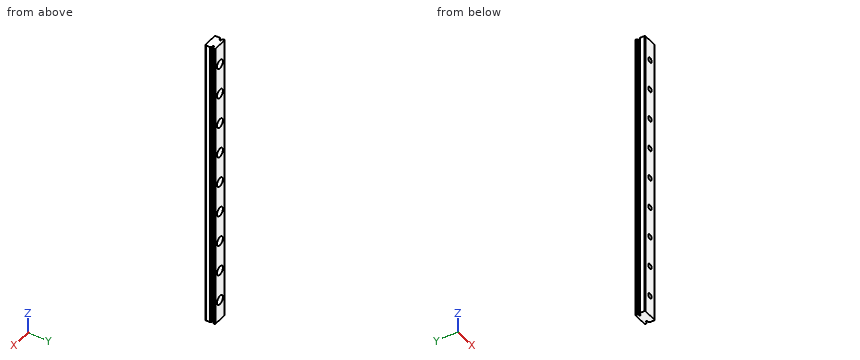
Autodesk Inventor part; units mm, degrees
ref_plane "to_block_XY" through (0, 4.7, 35) normal (0, 0, -1) x (1, 0, 0)
ref_plane "to_block_YZ" through (0, 4.7, 35) normal (1, 0, 0) x (0, -1, 0)
ref_plane "to_block_ZX" through (0, 4.7, 35) normal (0, -1, 0) x (0, 0, -1)
sketch "Sketch_12" plane through (0, 0, 0) normal (0, 0, 1) x (1, 0, 0)
  line L0 (-3.5, 4.4) -> (-3.5, 4.0339)
  line L1 (-3.5, 4.0339) -> (-3.2695, 3.9008)
  arc A0 (-2.9324, 3.55) -> (-3.2695, 3.9008) centre (-3.707, 3.143) ccw
  line L2 (-2.9324, 3.55) -> (-2.2, 3.55)
  line L3 (-2.2, 3.55) -> (-2.2, 2.85)
  line L4 (-2.2, 2.85) -> (-2.9324, 2.85)
  arc A1 (-3.2695, 2.4992) -> (-2.9324, 2.85) centre (-3.707, 3.257) ccw
  line L5 (-3.2695, 2.4992) -> (-3.5, 2.3662)
  line L6 (-3.5, 2.3662) -> (-3.5, 0.3)
  line L7 (-3.5, 0.3) -> (-3.2, 0)
  line L8 (-3.2, 0) -> (3.2, 0)
  line L9 (3.2, 0) -> (3.5, 0.3)
  line L10 (3.5, 0.3) -> (3.5, 2.3662)
  line L11 (3.5, 2.3662) -> (3.2695, 2.4992)
  arc A2 (2.9324, 2.85) -> (3.2695, 2.4992) centre (3.707, 3.257) ccw
  line L12 (2.9324, 2.85) -> (2.2, 2.85)
  line L13 (2.2, 2.85) -> (2.2, 3.55)
  line L14 (2.2, 3.55) -> (2.9324, 3.55)
  arc A3 (3.2695, 3.9008) -> (2.9324, 3.55) centre (3.707, 3.143) ccw
  line L15 (3.2695, 3.9008) -> (3.5, 4.0339)
  line L16 (3.5, 4.0339) -> (3.5, 4.4)
  line L17 (3.5, 4.4) -> (3.2, 4.7)
  line L18 (3.2, 4.7) -> (-3.2, 4.7)
  line L19 (-3.2, 4.7) -> (-3.5, 4.4)
extrude "Extrusion1" add sketch "Sketch_12" along normal mid plane 140
sketch "Sketch2" plane through (-3.2, 4.7, 70) normal (0, 1, 0) x (1, 0, 0)
  point P0 (3.2, 130)
hole "Hole1" at (0, 4.7, -60) direction (0, -1, 0) diameter 2.4 depth 4.7 counterbore diameter 4.2 counterbore depth 2.3
pattern_linear "Rectangular Pattern1" count 9 spacing 15 along (0, 0, 1) of "Hole1"
ref_plane "to_block_XY" through (0, 4.7, 35) normal (0, 0, -1) x (1, 0, 0)
ref_plane "to_block_YZ" through (0, 4.7, 35) normal (1, 0, 0) x (0, -1, 0)
ref_plane "to_block_ZX" through (0, 4.7, 35) normal (0, -1, 0) x (0, 0, -1)
ref_plane "to_block_2_XY" through (0, 4.7, -35) normal (0, 0, -1) x (1, 0, 0)
ref_plane "to_block_2_YZ" through (0, 4.7, -35) normal (1, 0, 0) x (0, -1, 0)
ref_plane "to_block_2_ZX" through (0, 4.7, -35) normal (0, -1, 0) x (0, 0, -1)
ref_plane "to_bolt_1_XY" through (0, 2.4, 60) normal (0, 1, 0) x (1, 0, 0)
ref_plane "to_bolt_1_YZ" through (0, 2.4, 60) normal (1, 0, 0) x (0, 0, -1)
ref_plane "to_bolt_1_ZX" through (0, 2.4, 60) normal (0, 0, -1) x (0, 1, 0)
ref_plane "to_bolt_2_XY" through (0, 2.4, 45) normal (0, 1, 0) x (1, 0, 0)
ref_plane "to_bolt_2_YZ" through (0, 2.4, 45) normal (1, 0, 0) x (0, 0, -1)
ref_plane "to_bolt_2_ZX" through (0, 2.4, 45) normal (0, 0, -1) x (0, 1, 0)
ref_plane "to_bolt_3_XY" through (0, 2.4, 30) normal (0, 1, 0) x (1, 0, 0)
ref_plane "to_bolt_3_YZ" through (0, 2.4, 30) normal (1, 0, 0) x (0, 0, -1)
ref_plane "to_bolt_3_ZX" through (0, 2.4, 30) normal (0, 0, -1) x (0, 1, 0)
ref_plane "to_bolt_4_XY" through (0, 2.4, 15) normal (0, 1, 0) x (1, 0, 0)
ref_plane "to_bolt_4_YZ" through (0, 2.4, 15) normal (1, 0, 0) x (0, 0, -1)
ref_plane "to_bolt_4_ZX" through (0, 2.4, 15) normal (0, 0, -1) x (0, 1, 0)
ref_plane "to_bolt_5_XY" through (0, 2.4, 0) normal (0, 1, 0) x (1, 0, 0)
ref_plane "to_bolt_5_YZ" through (0, 2.4, 0) normal (1, 0, 0) x (0, 0, -1)
ref_plane "to_bolt_5_ZX" through (0, 2.4, 0) normal (0, 0, -1) x (0, 1, 0)
ref_plane "to_bolt_6_XY" through (0, 2.4, -15) normal (0, 1, 0) x (1, 0, 0)
ref_plane "to_bolt_6_YZ" through (0, 2.4, -15) normal (1, 0, 0) x (0, 0, -1)
ref_plane "to_bolt_6_ZX" through (0, 2.4, -15) normal (0, 0, -1) x (0, 1, 0)
ref_plane "to_bolt_7_XY" through (0, 2.4, -30) normal (0, 1, 0) x (1, 0, 0)
ref_plane "to_bolt_7_YZ" through (0, 2.4, -30) normal (1, 0, 0) x (0, 0, -1)
ref_plane "to_bolt_7_ZX" through (0, 2.4, -30) normal (0, 0, -1) x (0, 1, 0)
ref_plane "to_bolt_8_XY" through (0, 2.4, -45) normal (0, 1, 0) x (1, 0, 0)
ref_plane "to_bolt_8_YZ" through (0, 2.4, -45) normal (1, 0, 0) x (0, 0, -1)
ref_plane "to_bolt_8_ZX" through (0, 2.4, -45) normal (0, 0, -1) x (0, 1, 0)
ref_plane "to_bolt_9_XY" through (0, 2.4, -60) normal (0, 1, 0) x (1, 0, 0)
ref_plane "to_bolt_9_YZ" through (0, 2.4, -60) normal (1, 0, 0) x (0, 0, -1)
ref_plane "to_bolt_9_ZX" through (0, 2.4, -60) normal (0, 0, -1) x (0, 1, 0)
properties part number "SSE2BLZ8-140_r1" material "ステンレス鋼"
CAD build for the part. Positions are in the model's coordinates, mm. Round coordinates to 2 decimals unless told otherwise and drop trailing zeros. Order: outer loops, then holes, each group sorted by start corner. A loop starts at its lowest first (then second) coordinate and runs counter-clockwise, first axis right, second up.
Q1. Slice it at C-C (y = 1.45). State how many separate pieces and enclosed holes the cut face has, and give its area (3 significant figures).
Q2. Wall check: L1, parallel to Y at x = -2.25, z = 26; L2, parallel to X at y = 0.95, z = 45; L3, parallel to Y at x = 3, z = 53. Give the ranges that are in metal, low to high.
Q3. Drop a flat-ended pin along its axis: pin 1 (3.5 mm diameter, centred on x = 0, z = -45, fed in from +Y). Give the stop position or say it passes through.
Q4. Slice it at B-B (z = 5.5). Write the cut outline in (x, y), and give its area (3 significant figures).
Results below:
1. separate pieces: 1
1. enclosed holes: 9
1. area: 939 mm2
2. L1: y = 0 to 2.85, 3.55 to 4.7
2. L2: x = -3.5 to -1.2, 1.2 to 3.5
2. L3: y = 0 to 2.74, 3.66 to 4.7
3. pin 1: stops at y = 2.4
4. outline: (-3.5, 0.3) - (-3.2, 0) - (3.2, 0) - (3.5, 0.3) - (3.5, 2.37) - (3.27, 2.5) arc R0.88 cw to (2.93, 2.85) - (2.2, 2.85) - (2.2, 3.55) - (2.93, 3.55) arc R0.87 cw to (3.27, 3.9) - (3.5, 4.03) - (3.5, 4.4) - (3.2, 4.7) - (-3.2, 4.7) - (-3.5, 4.4) - (-3.5, 4.03) - (-3.27, 3.9) arc R0.88 cw to (-2.93, 3.55) - (-2.2, 3.55) - (-2.2, 2.85) - (-2.93, 2.85) arc R0.87 cw to (-3.27, 2.5) - (-3.5, 2.37) - close
4. area: 30.2 mm2
